Verification items for the finished model (mm, model axes). A direction names the side the tool comes from. Give positions to 0.01 mm unless a question says otherwise; leave off trailing zeros. Order: outer loops, then holes, each group sorted by start corner. A loop starts at its lowest first (then second) coordinate and runs counter-clockwise, first axis right, second up.
from build123d import *

# Parameters (mm, degrees)
F0_W           = 148
F0_H           = 11.5
F1_DEPTH       = 2.5
F2_W           = 148
F2_H           = 20
F3_DEPTH       = 2
F5_D           = 6
F5_CSINK_D     = 11.7
F5_CSINK_ANGLE = 90
F6_R           = 5


with BuildPart() as f1:
    # F0 (on Front) → F1 (new body)
    with BuildSketch(Plane.XZ):
        with Locations((0, 5.75)):
            Rectangle(F0_W, F0_H)
    extrude(amount=-F1_DEPTH)

    # F2 (on face) → F3 (join)
    with BuildSketch(Plane(origin=(0, 2.5, 0), x_dir=(-1, 0, 0), z_dir=(0, 1, 0))):
        with Locations((0, 10)):
            Rectangle(F2_W, F2_H)
    extrude(amount=F3_DEPTH)

    # F5 (through all)
    with Locations(Plane(origin=(0, 4.5, 0), x_dir=(-1, 0, 0), z_dir=(0, 1, 0))):
        with Locations((-46, 5.75), (-6, 5.75), (34, 5.75)):
            CounterSinkHole(F5_D / 2, F5_CSINK_D / 2, counter_sink_angle=F5_CSINK_ANGLE)

    # F6
    f6_edges = [f1.edges().sort_by_distance(p)[0] for p in [
        (-74, 3.5, 20),
        (74, 3.5, 20),
    ]]
    fillet(f6_edges, radius=F6_R)


solid = f1.part
(1) Set-up check for faces 5 (the flat face through (-1, 1, 11.5)), 6 (the cylindrical face through (-36.997, 0.813, 5.882)): record each of +Z, -Z, +X, -X, +Y, -Y from which the full face is reachable in a straight line by a thin tool's end or side.
Solved:
face 5: +Z, +X, -X, -Y
face 6: +Y, -Y
(2) Scan lines: line 1 (X direction, y = 0.45, z = 5.75); line 2 (Z direction, x = 46, y = 1.1); line 3 (X direction, y = 1.5, z = 8.25). Record each from-to range of solid material in increasing order.
Solved:
line 1: x = -74 to -37, -31 to 3, 9 to 43, 49 to 74
line 2: z = 0 to 2.75, 8.75 to 11.5
line 3: x = -74 to -35.66, -32.34 to 4.34, 7.66 to 44.34, 47.66 to 74
(3) Go/stop test with a flat-tipped pin: pin 1 (2.5 mm diameter, centred on x = -16.5, z = 16.5, fed in from -Y). Record where the tip stops, or that it passes through.
Solved:
pin 1: stops at y = 2.5
(4) Section check B-B, the plane x = -52.5. Enter the section's corners in (y, z), then the cut area to 4 significant figures.
Solved:
outline: (0, 0) - (4.5, 0) - (4.5, 20) - (2.5, 20) - (2.5, 11.5) - (0, 11.5) - close
area: 68.75 mm2
(5) Release check for a two-part mould opening along X. For faces 1 (the cylindrical face through (7.384, 0.813, 3.088)), 2 (the flat face through (1, 4.5, 10)), 3 (the flat face through (-74, 2, 7)), 4 (the cylindrical face through (73, 4, 18)) record: pulls with the +X half, pulls with the -X half, needs draft (parallel to the pull), parting line crosses it, or undercut.
Solved:
face 1: undercut
face 2: needs draft
face 3: pulls with the -X half
face 4: pulls with the +X half
(6) Section check C-C, the plane z = 17. Enter the section's corners in (x, y), then the cut area to 3 significant figures.
Solved:
outline: (-73.58, 2.5) - (73.58, 2.5) - (73.58, 4.5) - (-73.58, 4.5) - close
area: 294 mm2
(7) Section check A-A, the plane z = 5.75. Enter the section's corners in (x, y).
Solved:
outline: (-74, 0) - (-37, 0) - (-37, 1.65) - (-39.85, 4.5) - (-74, 4.5) - close; (-31, 0) - (3, 0) - (3, 1.65) - (0.15, 4.5) - (-28.15, 4.5) - (-31, 1.65) - close; (9, 0) - (43, 0) - (43, 1.65) - (40.15, 4.5) - (11.85, 4.5) - (9, 1.65) - close; (49, 0) - (74, 0) - (74, 4.5) - (51.85, 4.5) - (49, 1.65) - close
